```python
from build123d import *

# Parameters (mm, degrees)
F1_DEPTH = 50
F2_SIZE2 = 10
F2_SIZE  = 58
F3_SIZE2 = 62
F3_SIZE  = 10


with BuildPart() as f1:
    # F0 (on Right) → F1 (new body)
    with BuildSketch(Plane.YZ):
        Polygon((482.7914457609, 377.3975717771), (463.0650614387, 400), (163.0650614387, 400), (86.8967218104, 1020.3413447758), (66.1366664017, 1041.9982166512), (11.6469021237, 976.7612210971), (92.2870402742, 320), (452.2870402742, 320), align=None)
    extrude(amount=-F1_DEPTH)

    # F2
    f2_edges = [f1.edges().sort_by_distance(p)[0] for p in [
        (-50, 272.28704, 320),
    ]]
    f2_side = f1.faces().sort_by_distance((-50, 466.432885, 383.02992))[0]
    chamfer(f2_edges, length=F2_SIZE, length2=F2_SIZE2, reference=f2_side)

    # F3
    f3_edges = [f1.edges().sort_by_distance(p)[0] for p in [
        (-50, 48.406219, 677.380611),
    ]]
    f3_side = f1.faces().sort_by_distance((-24.806952, 51.628874, 651.134191))[0]
    chamfer(f3_edges, length=F3_SIZE, length2=F3_SIZE2, reference=f3_side)


solid = f1.part
```
CAD build for the part. Positions are in the model's coordinates, mm. A direction names the side the tool comes from. Round coordinates to 2 decimals unless told otherwise and drop trailing zeros. Loops run counter-clockwise (first coordinate to the right, second up) from the corner with the lowest first, then second, coordinate; pieces in that order, holes last. Notation, with made-up numbers: M 47.25,25 L 67.25,25 A29 ccw 67.25,61 Z; hole C -31.5,18 d10. An arc over 180 degrees is marked long. Use a Markdown table: item, result. Add a question column.
(1) Flat gauge pins, fed straight in: pin 1 (8 mm diameter, centred on x = -20, y = 338, fed in from +Z); pin 2 (5 mm diameter, centred on x = -32, z = 455.5, fed in from -Y); pin 3 (8 mm diameter, centred on x = -7.5, z = 583.5, fed in from +Y). Where does each tip first touch, or does it go through?
(2) Cut at A-A (x = -15). Give the cut face in (y, z).
(3) Cut at C-C (z = 987). Give the cut face in (x, y).
(4) Cut at B-B (y = 199.5). Give the cut face in (x, z).
(5) Drill centre lines: line 1 (Z direction, x = -33, y = 172.5); line 2 (X direction, y = 58.5, z = 819); line 3 (Y direction, x = -19.5, z = 371.5). Where is each one in solid material? Low to high.
(6) Cut at D-D (y = 101.5). Give the cut face in (x, z), and give its area (3 significant figures).
(7) Which spindle directions (+Z, -Z, +X, -X, +Y, -Y) get a long thin tool onto all of the face, cutting with end or side? Do faces 1 (the face through (0, 141, 576)), 2 (the face through (-25, 315, 400)). Say none if no direction does.
Geometry says:
| question | item | result |
|---|---|---|
| 1 | pin 1 | stops at z = 400 |
| 1 | pin 2 | stops at y = 75.34 |
| 1 | pin 3 | stops at y = 141.03 |
| 2 | outline | M 11.65,976.76 L 92.29,320 L 452.29,320 L 482.79,377.4 L 463.07,400 L 163.07,400 L 86.9,1020.34 L 66.14,1042 Z |
| 3 | outline | M -50,72.86 L -41.57,20.2 L 0,20.2 L 0,90.99 L -50,90.99 Z |
| 4 | outline | M -50,378 L -40,320 L 0,320 L 0,400 L -50,400 Z |
| 5 | line 1 | z = 320 to 400 |
| 5 | line 2 | x = -44.4 to 0 |
| 5 | line 3 | y = 85.96 to 479.66 |
| 6 | outline | M -50,753.71 L -41.66,329.66 L -40,320 L 0,320 L 0,901.41 L -50,901.41 Z |
| 6 | area | 27,200 mm² |
| 7 | face 1 | +Z, -Z, +X, +Y, -Y |
| 7 | face 2 | +Z, +X, -X, +Y |
